CAD build for the part. Positions are in the model's coordinates, mm. Face numbers are marked on the shaded views. A direction names the side the tool comes from. Round coordinates to 2 decimals unless told otherwise and drop trailing zeros. Order: outer loops, then holes, each group sorted by start corner. A loop starts at its lowest first (then second) coordinate and runs counter-clockwise, first axis right, second up. Notation, with made-up numbers: (81, 36) -> (100, 36) arc R31 cw to (100, 74) -> close; hole circle Ø3 at (73, 62.5). An arc over 180 degrees is marked (long way). Return JSON: item names as keys, results as strings. Group by question number.
Q1. Cut at D-D (x = -8). Write the cut outline in (y, z), then the cut area to 3 significant figures.
Q2. Which spindle directions (+Z, -Z, +X, -X, +Y, -Y) get a long thin tool onto all of the face, cutting with end or side? Do the marked faces 1 and 2. Say none if no direction does.
Q3. Probe line 1 along Z through (x, y) = (0.25, 12); line 2 along X through (y, z) = (18.5, 0.75); line 3 along X through (y, z) = (14, 4.75). List the from-to ranges inside material, lowest first.
Q4. Mould opens along X. For the marked faces 3, 4 and 5 say: +X half, -X half, draft (parallel to the pull), parting line (faces both ways), or undercut.
Q5. Flat gauge pins, fed straight in: pin 1 (4 mm diameter, centred on y = 8.5, z = -8, fed in from +X); pin 2 (1.5 mm diameter, centred on y = 19, z = -6, fed in from +X); pin 3 (1 mm diameter, centred on y = 23, z = -2.5, fed in from -X). Where does each tip first touch, or does it go through?
Q6. Cut at B-B (x = 0). Write the cut outline in (y, z).
Q7. Cut at C-C (z = 4.75). Write the cut outline in (x, y), then the cut area to 3 significant figures.
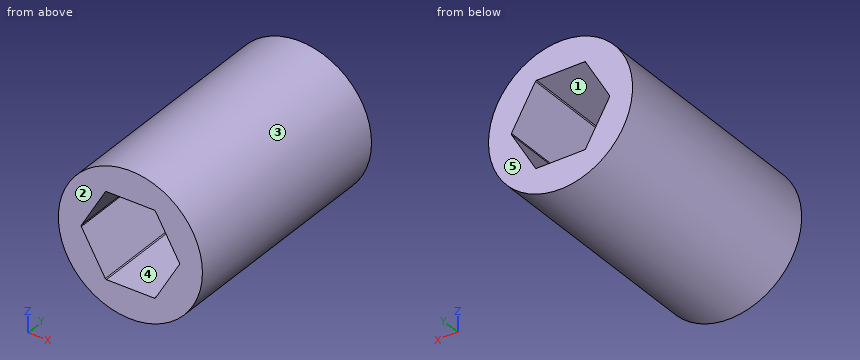
from build123d import *

# Parameters (mm, degrees)
SKETCH1_R           = 11.1125
BOSS_EXTRUDE1_DEPTH = 36.7538
FILLET1_R           = 0.2


with BuildPart() as part:
    # Sketch1 → Boss-Extrude1 (new body)
    with BuildSketch(Plane(origin=(0, 0, 0), x_dir=(1, 0, 0), z_dir=(0, 1, 0))):
        Circle(SKETCH1_R)
        Polygon((7.625642355, 0), (3.812821178, 6.604), (-3.812821178, 6.604), (-7.625642355, 0), (-3.812821178, -6.604), (3.812821178, -6.604), align=None, mode=Mode.SUBTRACT)
    extrude(amount=BOSS_EXTRUDE1_DEPTH)

    # Fillet1
    fillet1_edges = [part.edges().sort_by_distance(p)[0] for p in [
        (7.625642355, 18.3769, 0),
        (3.812821178, 18.3769, -6.604),
        (-3.812821178, 18.3769, -6.604),
        (-7.625642355, 18.3769, 0),
        (-3.812821178, 18.3769, 6.604),
        (3.812821178, 18.3769, 6.604),
    ]]
    fillet(fillet1_edges, radius=FILLET1_R)


solid = part.part
Solution:
{
 "1": {"outline": "(0, -7.71) -> (36.75, -7.71) -> (36.75, 7.71) -> (0, 7.71) -> close", "area": "567 mm²"},
 "2": {"face 1": "+Y, -Y", "face 2": "+Z, -Z, +X, -X, -Y"},
 "3": {"line 1": "z = -11.11 to -6.6, 6.6 to 11.11", "line 2": "x = -11.09 to -7.19, 7.19 to 11.09", "line 3": "x = -10.05 to -4.88, 4.88 to 10.05"},
 "4": {"face 3": "parting line", "face 4": "undercut", "face 5": "draft"},
 "5": {"pin 1": "stops at x = 9.35", "pin 2": "stops at x = 9.79", "pin 3": "stops at x = -10.93"},
 "6": {"outline": "(0, -11.11) -> (36.75, -11.11) -> (36.75, -6.6) -> (0, -6.6) -> close; (0, 6.6) -> (36.75, 6.6) -> (36.75, 11.11) -> (0, 11.11) -> close"},
 "7": {"outline": "(-10.05, 0) -> (-4.88, 0) -> (-4.88, 36.75) -> (-10.05, 36.75) -> close; (4.88, 0) -> (10.05, 0) -> (10.05, 36.75) -> (4.88, 36.75) -> close", "area": "380 mm²"}
}
